For this review, take the finished solid that the model builds, in its own axes (mm). A direction names the side the tool comes from. Coordinates: 2 decimals unless noted, no trailing zeros. Order: outer loops, then holes, each group sorted by start corner. A loop starts at its lowest first (then second) coordinate and runs counter-clockwise, first axis right, second up. Notation, with made-up numbers: (80.25, 86.5) - (121.25, 86.5) arc R22 cw to (121.25, 105.5) - close; hole circle Ø4 at (57.5, 58). An arc over 180 degrees is marked (long way). One line per item, written item: value. Start each with the question number.
(1) Clearance check with flat-ended pins moving along their axes: pin 1 (12 mm diameter, centred on x = 6.5, z = 6, fed in from +Y); pin 2 (2.5 mm diameter, centred on x = -1, y = -2.5, fed in from +Z); pin 3 (6.5 mm diameter, centred on x = -0.5, y = -4, fed in from -Z). State where each tip first meets the part, or that it passes through.
(2) To check wall thickness, follow line 1 along X through (y, z) = (-49, -2.5); line 2 along Z through (x, y) = (5, -56); line 3 along Y through (x, z) = (0, 5). State the ranges of each line that lie inside material, in increasing order.
(3) Consider section A-A on y = 0. Write out the cut boundary in (x, z).
(4) Consider section C-C on z = 12. Write out the cut boundary in (x, y), then the cut area to 3 significant figures.
(5) For faces 4 (the flat face through (1, -4, 0)), 5 (the cylindrical face through (0.25, -24.53, 5.98)), 6 (the flat face through (0, -21, -1.119)), list the 3-axis set-ups (+Z, -Z, +X, -X, +Y, -Y) from which the entire face can be reached by the end or side of a thin tool; tool diameter is ignored.
(6) Mouldability with a two-part tool opening along X and no side actions: class faces 1 (the flat face through (0, -17, -7)), 2 (the flat face through (-0.1, -19.109, 8.6)), 3 (the cylindrical face through (0, 4, 3)) as released by +X, released by -X, zero draft, split by the parting line, or undercut.
(7) Consider section B-B on y = -26. Count the separate pieces of the cut face and the enclosed holes in it, then the cut area to 3 significant figures.
```python
from build123d import *

# Parameters (mm, degrees)
SKETCH2_R                = 4
SKETCH2_R_2              = 3
BOSS_EXTRUDE1_DEPTH      = 7
BOSS_EXTRUDE2_DEPTH      = 7
BOSS_EXTRUDE3_DEPTH      = 7
BOSS_EXTRUDE3_DEPTH_BACK = 14
SKETCH5_W                = 2.481427535
SKETCH5_H                = 11.249138159
SKETCH5_W_2              = 2.867427374
SKETCH5_W_3              = 2.922570208
CUT_EXTRUDE2_DEPTH       = 169
CUT_EXTRUDE2_DEPTH_BACK  = 169
SKETCH6_R                = 1
BOSS_EXTRUDE5_DEPTH      = 60


with BuildPart() as part:
    # Sketch2 → Boss-Extrude1 (new body)
    with BuildSketch(Plane.XY):
        Circle(SKETCH2_R)
        Circle(SKETCH2_R_2, mode=Mode.SUBTRACT)
    extrude(amount=BOSS_EXTRUDE1_DEPTH)

    # Sketch3 → Boss-Extrude2 (add)
    with BuildSketch(Plane.XY.offset(7)):
        Polygon((0, -3), (-1.5, -3), (-1.5, -13), (1.5, -13), (1.5, -3), align=None)
    extrude(amount=-BOSS_EXTRUDE2_DEPTH)

    # Sketch4 → Boss-Extrude3 (add, two sides)
    with BuildSketch(Plane.XY.offset(7)) as boss_extrude3_sk:
        with BuildLine():
            Line((1.5, -13), (11.531332628, -13))
            ThreePointArc((11.531332628, -13), (0, -24.531332628), (-11.531332628, -13))
            Line((-11.531332628, -13), (-1.5, -13))
            Line((-1.5, -13), (1.5, -13))
        make_face()
    extrude(amount=BOSS_EXTRUDE3_DEPTH)
    extrude(boss_extrude3_sk.sketch, amount=-BOSS_EXTRUDE3_DEPTH_BACK)

    # Sketch5 → Cut-Extrude2 (cut, two sides)
    with BuildSketch(Plane(origin=(1.5, 0, 0), x_dir=(0, 0, -1), z_dir=(1, 0, 0))) as cut_extrude2_sk:
        with Locations((-9.661011409, -24.733382447)):
            Rectangle(SKETCH5_W, SKETCH5_H)
        with Locations((-3.84344241, -24.733382447)):
            Rectangle(SKETCH5_W_2, SKETCH5_H)
        with Locations((2.580697764, -24.733382447)):
            Rectangle(SKETCH5_W_3, SKETCH5_H)
    extrude(amount=CUT_EXTRUDE2_DEPTH, mode=Mode.SUBTRACT)
    extrude(cut_extrude2_sk.sketch, amount=-CUT_EXTRUDE2_DEPTH_BACK, mode=Mode.SUBTRACT)

    # Sketch6 → Boss-Extrude5 (add)
    with BuildSketch(Plane.XZ.offset(19.108813367)):
        with Locations((-5.486205248, 9.734324146)):
            Circle(SKETCH6_R)
        with Locations((-0.486205248, 9.734324146)):
            Circle(SKETCH6_R)
        with Locations((4.513794752, 9.734324146)):
            Circle(SKETCH6_R)
        with Locations((-0.486205248, 3.634324146)):
            Circle(SKETCH6_R)
        with Locations((4.513794752, 3.634324146)):
            Circle(SKETCH6_R)
        with Locations((-0.486205248, -2.465675854)):
            Circle(SKETCH6_R)
        with Locations((4.513794752, -2.465675854)):
            Circle(SKETCH6_R)
        with Locations((-5.486205248, 3.634324146)):
            Circle(SKETCH6_R)
        with Locations((-5.486205248, -2.465675854)):
            Circle(SKETCH6_R)
    extrude(amount=BOSS_EXTRUDE5_DEPTH)


solid = part.part
```
Geometry check:
1. pin 1: stops at y = 3.97
1. pin 2: stops at z = 7
1. pin 3: stops at z = 0
2. line 1: x = -6.49 to -4.49, -1.49 to 0.51, 3.51 to 5.51
2. line 2: z = -3.34 to -1.59, 2.76 to 4.51, 8.86 to 10.61
2. line 3: y = -19.11 to -3, 3 to 4
3. outline: (-4, 0) - (-3, 0) - (-3, 7) - (-4, 7) - close; (3, 0) - (4, 0) - (4, 7) - (3, 7) - close
4. outline: (-11.53, -13) arc R11.53 ccw to (11.53, -13) - close
4. area: 209 mm^2
5. face 4: -Z, +X, -X, +Y
5. face 5: -Y
5. face 6: +X, -X, -Y
6. face 1: zero draft
6. face 2: undercut
6. face 3: split by the parting line
7. separate pieces: 9
7. enclosed holes: 0
7. area: 28.3 mm^2
